from build123d import *

# Parameters (mm, degrees)
BOSS_EXTRUDE1_DEPTH = 0.762
SKETCH3_R           = 1.1557
BOSS_EXTRUDE2_DEPTH = 3.937
CHAMFER1_SIZE       = 0.1


with BuildPart() as part:
    # Sketch2 → Boss-Extrude1 (new body)
    with BuildSketch(Plane(origin=(0, 0, 0), x_dir=(1, 0, 0), z_dir=(0, 1, 0))):
        with BuildLine():
            ThreePointArc((-2.886363636, 1.62557376), (-4.826, 0), (-2.886363636, -1.62557376))
            ThreePointArc((-2.886363636, -1.62557376), (0, -1.371311361), (2.886363636, -1.62557376))
            ThreePointArc((2.886363636, -1.62557376), (4.826, 0), (2.886363636, 1.62557376))
            ThreePointArc((2.886363636, 1.62557376), (0, 1.371311361), (-2.886363636, 1.62557376))
        make_face()
    extrude(amount=BOSS_EXTRUDE1_DEPTH)

    # Sketch3 → Boss-Extrude2 (add)
    with BuildSketch(Plane(origin=(0, 0.762, 0), x_dir=(1, 0, 0), z_dir=(0, 1, 0))):
        with Locations(Location((-3.175, 0, 0), (0, 0, 270))):
            Circle(SKETCH3_R)
        with Locations(Location((3.175, 0, 0), (0, 0, 270))):
            Circle(SKETCH3_R)
    extrude(amount=BOSS_EXTRUDE2_DEPTH)

    # Chamfer1
    chamfer1_edges = [part.edges().sort_by_distance(p)[0] for p in [
        (-3.175, 4.699, -1.1557),
        (3.175, 4.699, -1.1557),
    ]]
    chamfer(chamfer1_edges, length=CHAMFER1_SIZE)


solid = part.part
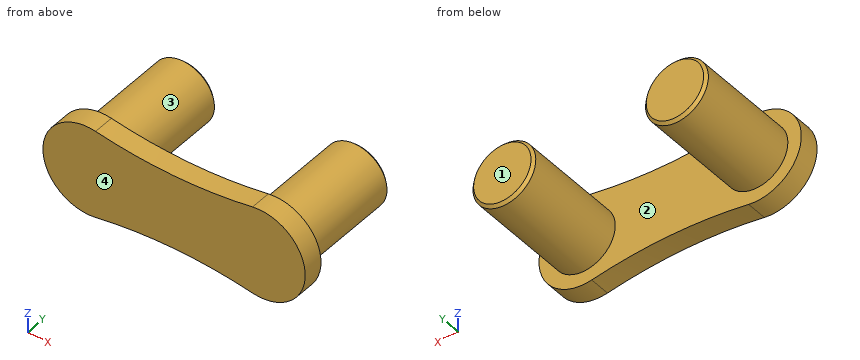
Here's how the part is built. I have some questions about the finished solid (model axes, mm). Face numbers are marked on the shaded views. A direction names the side the tool comes from. Coordinates: 2 decimals unless noted, no trailing zeros. Write each loop counter-clockwise with the first axis right and the second up, starting at its lowest first coordinate (ties: lowest second). Pieces come first, ordered by that corner, then holes.
1) If we section it at A-A (z = 0): List the corners of the cut face in (x, y) for me.
Filled in:
outline: (-4.83, 0) - (4.83, 0) - (4.83, 0.76) - (4.33, 0.76) - (4.33, 4.6) - (4.23, 4.7) - (2.12, 4.7) - (2.02, 4.6) - (2.02, 0.76) - (-2.02, 0.76) - (-2.02, 4.6) - (-2.12, 4.7) - (-4.23, 4.7) - (-4.33, 4.6) - (-4.33, 0.76) - (-4.83, 0.76) - close
2) If we section it at C-C (y = 2.75): List the corners of the cut face in (x, z) for me (3 decimals).
Filled in:
outline: circle Ø2.311 at (-3.175, 0); circle Ø2.311 at (3.175, 0)
3) If we section it at B-B (y = 0.5): List the corners of the cut face in (x, z) for me (3 decimals), plus the area to 3 significant figures.
Filled in:
outline: (-2.886, -1.626) arc R16.51 cw to (2.886, -1.626) arc R1.651 ccw (long way) to (2.886, 1.626) arc R16.51 cw to (-2.886, 1.626) arc R1.651 ccw (long way) to start
area: 27.3 mm2
4) I'm going to push a flat-ended pin straight in: pin 1 (2 mm diameter, centred on x = 3.5, y = 1.5, fed in from +Z). Where does the tip first touch, or does it pass through?
Filled in:
pin 1: stops at z = 1.65
5) If we section it at D-D (x = 0): List the corners of the cut face in (y, z) for me.
Filled in:
outline: (0, -1.37) - (0.76, -1.37) - (0.76, 1.37) - (0, 1.37) - close
6) If I drill on line 1 (Y direction, x = 2, z = 0.95); line 2 (X direction, y = 1.2, z = -0.1); line 3 (X direction, y = 4.35, z = 0.55), over which ranges is the centre line in solid material (lowest first)?
Filled in:
line 1: y = 0 to 0.76
line 2: x = -4.33 to -2.02, 2.02 to 4.33
line 3: x = -4.19 to -2.16, 2.16 to 4.19
7) Thinking about a two-plate mould opening in X: for the marked faces 3 and 4, which applies, +X half, -X half, draft (parallel to the pull), parting line (faces both ways), or undercut?
Filled in:
face 3: undercut
face 4: draft
8) Which directions (+Z, -Z, +X, -X, +Y, -Y) give clear straight access to the entire face, cutting with the end or side of a thin tool? Please do the marked faces 1 and 2.
Filled in:
face 1: +Z, -Z, +X, -X, +Y
face 2: +Y
